The model under review builds one solid part; all positions refer to its coordinate system, in mm. Face numbers are marked on the shaded views. A direction names the side the tool comes from. Round coordinates to 2 decimals unless told otherwise and drop trailing zeros. Write each loop counter-clockwise with the first axis right and the second up, starting at its lowest first coordinate (ties: lowest second). Pieces come first, ordered by that corner, then holes.
Item 1: Clearance check with flat-ended pins moving along their axes: pin 1 Ø9 at (x, y) = (62.5, 0) entering from +Z; pin 2 Ø6 at (x, z) = (35, 7) entering from +Y; pin 3 Ø5 at (x, z) = (-6.5, 13) entering from +Y; pin 4 Ø7 at (x, y) = (-44.19, -44.19) entering from -Z. State where each tip first meets the part, or that it passes through.
Item 2: To check wall thickness, follow L1, parallel to X at y = 0, z = 15.75; L2, parallel to X at y = 44, z = 7; L3, parallel to X at y = 40.5, z = 0.25. State the ranges of each line that lie inside material, in increasing order.
Item 3: Add section D-D (x = -19). Give the boundary of the cut face in (y, z).
Item 4: Add section A-A (y = 0). Give the boundary of the cut face in (x, z), plus the area to 3 significant figures.
Item 5: Draft analysis for pull direction Y (two halves, no side actions). For the marked faces 4, 5 and 6, state which applies: +Y half, -Y half, draft (parallel to the pull), parting line (faces both ways), or undercut.
Item 6: Machinability: for the marked faces 1, 2 and 3, which of the approach directions +Z, -Z, +X, -X, +Y, -Y give a long, thin tool a straight path to every point of the face, cutting with its end or side? Answer none if there is none.
Item 7: Add section B-B (y = -36). Give the boundary of the cut face in (x, z), plus the area to 3 significant figures.
Item 8: Add section C-C (z = -7). Give the boundary of the cut face in (x, y).
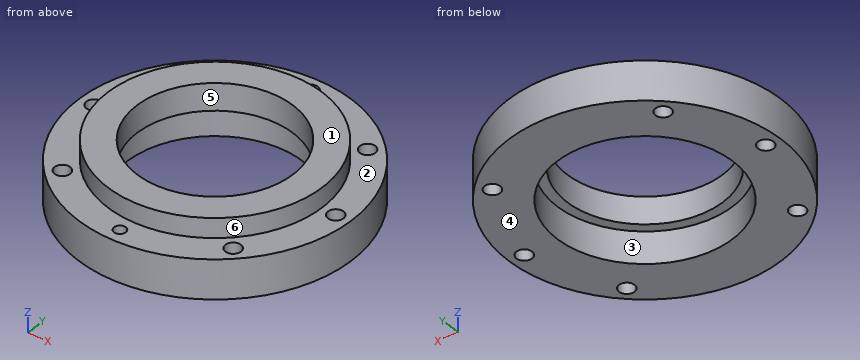
```python
from build123d import *

# Parameters (mm, degrees)
SKETCH2_R             = 3
CUT_EXTRUDE1_DEPTH    = 9
SKETCH3_R             = 4
CUT_EXTRUDE2_DEPTH    = 10
F_8_0MM_DOWEL_HOLE1_D = 8


with BuildPart() as part:
    # Sketch1 → Revolve1 (revolve)
    with BuildSketch(Plane(origin=(0, 0, 0), x_dir=(1, 0, 0), z_dir=(0, 1, 0))):
        Polygon((-55, -19.79575879), (-55, -9.79575879), (-70, -9.79575879), (-70, 10.20424121), (-45, 10.20424121), (-45, -6), (-40, -6), (-40, -19.79575879), align=None)
    revolve(axis=Axis((0, 0, -52.707374268), (0, 0, 1)))

    # Sketch2 → Cut-Extrude1 (cut)
    with BuildSketch(Plane.XY.offset(9.79575879)):
        with Locations((0, -62.5)):
            Circle(SKETCH2_R)
    extrude(amount=-CUT_EXTRUDE1_DEPTH, mode=Mode.SUBTRACT)

    # Sketch3 → Cut-Extrude2 (cut)
    with BuildSketch(Plane.XY.offset(9.79575879)):
        with Locations((0, 62.5)):
            Circle(SKETCH3_R)
    extrude(amount=-CUT_EXTRUDE2_DEPTH, mode=Mode.SUBTRACT)

    # Ø8.0mm Dowel Hole1 (through all)
    with Locations(Plane.XY.offset(9.79575879)):
        with Locations((44.194173824, 44.194173824), (62.5, 0), (44.194173824, -44.194173824), (-44.194173824, -44.194173824), (-62.5, 0), (-44.194173824, 44.194173824)):
            Hole(F_8_0MM_DOWEL_HOLE1_D / 2)


solid = part.part
```
Numbers:
1. pin 1: stops at z = 9.8
1. pin 2: stops at y = 62.26
1. pin 3: stops at y = 54.85
1. pin 4: passes through
2. L1: x = -55 to -40, 40 to 55
2. L2: x = -54.44 to -48.19, -40.2 to 40.2, 48.19 to 54.44
2. L3: x = -57.09 to -45.73, -42.66 to -19.62, 19.62 to 42.66, 45.73 to 57.09
3. outline: (-67.37, -10.2) - (-40.79, -10.2) - (-40.79, 6) - (-35.2, 6) - (-35.2, 19.8) - (-51.61, 19.8) - (-51.61, 9.8) - (-67.37, 9.8) - close; (35.2, 6) - (40.79, 6) - (40.79, -10.2) - (67.37, -10.2) - (67.37, 9.8) - (51.61, 9.8) - (51.61, 19.8) - (35.2, 19.8) - close
4. outline: (-70, -10.2) - (-66.5, -10.2) - (-66.5, 9.8) - (-70, 9.8) - close; (-58.5, -10.2) - (-45, -10.2) - (-45, 6) - (-40, 6) - (-40, 19.8) - (-55, 19.8) - (-55, 9.8) - (-58.5, 9.8) - close; (40, 6) - (45, 6) - (45, -10.2) - (58.5, -10.2) - (58.5, 9.8) - (55, 9.8) - (55, 19.8) - (40, 19.8) - close; (66.5, -10.2) - (70, -10.2) - (70, 9.8) - (66.5, 9.8) - close
4. area: 1,020 mm2
5. face 4: draft
5. face 5: undercut
5. face 6: parting line
6. face 1: +Z, +X, -X, +Y, -Y
6. face 2: +Z
6. face 3: -Z
7. outline: (-60.03, -10.2) - (-27, -10.2) - (-27, 6) - (-17.44, 6) - (-17.44, 19.8) - (-41.58, 19.8) - (-41.58, 9.8) - (-60.03, 9.8) - close; (17.44, 6) - (27, 6) - (27, -10.2) - (60.03, -10.2) - (60.03, 9.8) - (41.58, 9.8) - (41.58, 19.8) - (17.44, 19.8) - close
7. area: 1,880 mm2
8. outline: circle Ø140 at (0, 0); hole circle Ø8 at (-62.5, 0); hole circle Ø8 at (-44.19, -44.19); hole circle Ø8 at (-44.19, 44.19); hole circle Ø90 at (0, 0); hole circle Ø8 at (44.19, -44.19); hole circle Ø8 at (44.19, 44.19); hole circle Ø8 at (62.5, 0)
